Read the model definition and answer for the solid it produces. Units are mm, in the model's axes. Coordinates: 2 decimals unless noted, no trailing zeros. Order: outer loops, then holes, each group sorted by start corner. A loop starts at its lowest first (then second) coordinate and runs counter-clockwise, first axis right, second up. Notation, with made-up numbers: (33.25, 87) - (79.25, 87) arc R23 cw to (79.25, 120) - close; hole circle Ø10 at (59.5, 84.5). An arc over 180 degrees is marked (long way). Use one line per item in the form item = value.
```python
from build123d import *

# Parameters (mm, degrees)
SKETCH1_W           = 7.87
SKETCH1_H           = 5.59
BOSS_EXTRUDE1_DEPTH = 5.13
BOSS_EXTRUDE1_TAPER = 1
SKETCH2_W           = 0.76
SKETCH2_H           = 1.16
BOSS_EXTRUDE2_DEPTH = 0.1
FILLET1_R           = 0.1
SKETCH3_R           = 0.4
CUT_EXTRUDE1_DEPTH  = 0.02


with BuildPart() as part:
    # Sketch1 → Boss-Extrude1 (new body)
    with BuildSketch(Plane(origin=(0, 0, 0), x_dir=(1, 0, 0), z_dir=(0, 1, 0))):
        Rectangle(SKETCH1_W, SKETCH1_H)
    extrude(amount=BOSS_EXTRUDE1_DEPTH, taper=BOSS_EXTRUDE1_TAPER)

    # Sketch2 → Boss-Extrude2 (add, symmetric)
    with BuildSketch(Plane.XZ):
        with Locations((0, 2.875)):
            Rectangle(SKETCH2_W, SKETCH2_H)
        with Locations((2.54, 2.875)):
            Rectangle(SKETCH2_W, SKETCH2_H)
        with Locations((-2.54, 2.875)):
            Rectangle(SKETCH2_W, SKETCH2_H)
        with Locations((-2.54, -2.875)):
            Rectangle(SKETCH2_W, SKETCH2_H)
        with Locations((0, -2.875)):
            Rectangle(SKETCH2_W, SKETCH2_H)
        with Locations((2.54, -2.875)):
            Rectangle(SKETCH2_W, SKETCH2_H)
    extrude(amount=BOSS_EXTRUDE2_DEPTH, both=True)

    # Fillet1
    fillet1_edges = [part.edges().sort_by_distance(p)[0] for p in [
        (2.92, 0, -3.455),
        (2.16, 0, -3.455),
        (-3.845455517, 5.13, 0),
        (0, 5.13, 2.705455517),
        (-0.38, 0, 3.455),
        (0.38, 0, 3.455),
        (-2.92, 0, 3.455),
        (-2.16, 0, 3.455),
        (3.845455517, 5.13, 0),
        (2.16, 0, 3.455),
        (2.92, 0, 3.455),
        (-2.16, 0, -3.455),
        (-2.92, 0, -3.455),
        (3.890227758, 2.565, 2.750227758),
        (-3.890227758, 2.565, 2.750227758),
        (-3.890227758, 2.565, -2.750227758),
        (3.890227758, 2.565, -2.750227758),
        (0.38, 0, -3.455),
        (-0.38, 0, -3.455),
        (0, 5.13, -2.705455517),
    ]]
    fillet(fillet1_edges, radius=FILLET1_R)

    # Sketch3 → Cut-Extrude1 (cut)
    with BuildSketch(Plane(origin=(0, 5.13, 0), x_dir=(1, 0, 0), z_dir=(0, 1, 0))):
        with Locations((-3.047185791, -1.907185791)):
            Circle(SKETCH3_R)
    extrude(amount=-CUT_EXTRUDE1_DEPTH, mode=Mode.SUBTRACT)


solid = part.part
```
(1) Straight lines are drawn through the part: L1, parallel to Y at x = 3, z = -1; L2, parallel to X at y = 4.95, z = -0.5; L3, parallel to Z at x = 3, y = 0.15. For each, find the intervals that lie inside material, in ascending order.
Answer list:
L1 = 0 to 5.13
L2 = -3.85 to 3.85
L3 = -2.79 to 2.79
(2) Given pin 1 Ø1 at (x, y) = (-1, 1) entering from -Z; pin 2 Ø1.5 at (x, y) = (3, 4.5) entering from +Z; pin 3 Ø0.5 at (x, z) = (0, -3.5) entering from +Y, each flat-ended and moving along its own axis, determine where each tip first touches the part or whether it passes through.
Answer list:
pin_1 = -2.79
pin_2 = 2.73
pin_3 = 0.1
(3) The mould has two halves that part along Z. Classify faces 1 (the flat face through (0, 5.13, 0)), 2 (the flat face through (0, 0, 0)): +Z half, -Z half, draft (parallel to the pull), parting line (faces both ways), or undercut.
Answer list:
face_1 = draft
face_2 = undercut
(4) Section A-A, the plane z = 3 is taken. Write down the section's boundary in (x, y), then the cut area to 3 significant figures.
Answer list:
outline = (-2.92, -0.1) - (-2.16, -0.1) - (-2.16, 0.1) - (-2.92, 0.1) - close; (-0.38, -0.1) - (0.38, -0.1) - (0.38, 0.1) - (-0.38, 0.1) - close; (2.16, -0.1) - (2.92, -0.1) - (2.92, 0.1) - (2.16, 0.1) - close
area = 0.456 mm2
